Check sheet for the drawn part. Datum: minimum x, y, z corner. Units: mm. A direction names the side the tool comes from. Round coordinates to 2 decimals unless told otherwise and drop trailing zeros. Write each loop counter-clockwise with the first axis right and the second up, starting at its lowest first coordinate (ties: lowest second). Pieces come first, ordered by that corner, then holes. Notation, with made-up numbers: (7.25, 39) - (43.25, 39) arc R17 ccw to (43.25, 63) - close; hole circle Ø3 at (37.5, -4.5). An arc over 180 degrees is marked (long way). Answer as a JSON object with one key per item and string values.
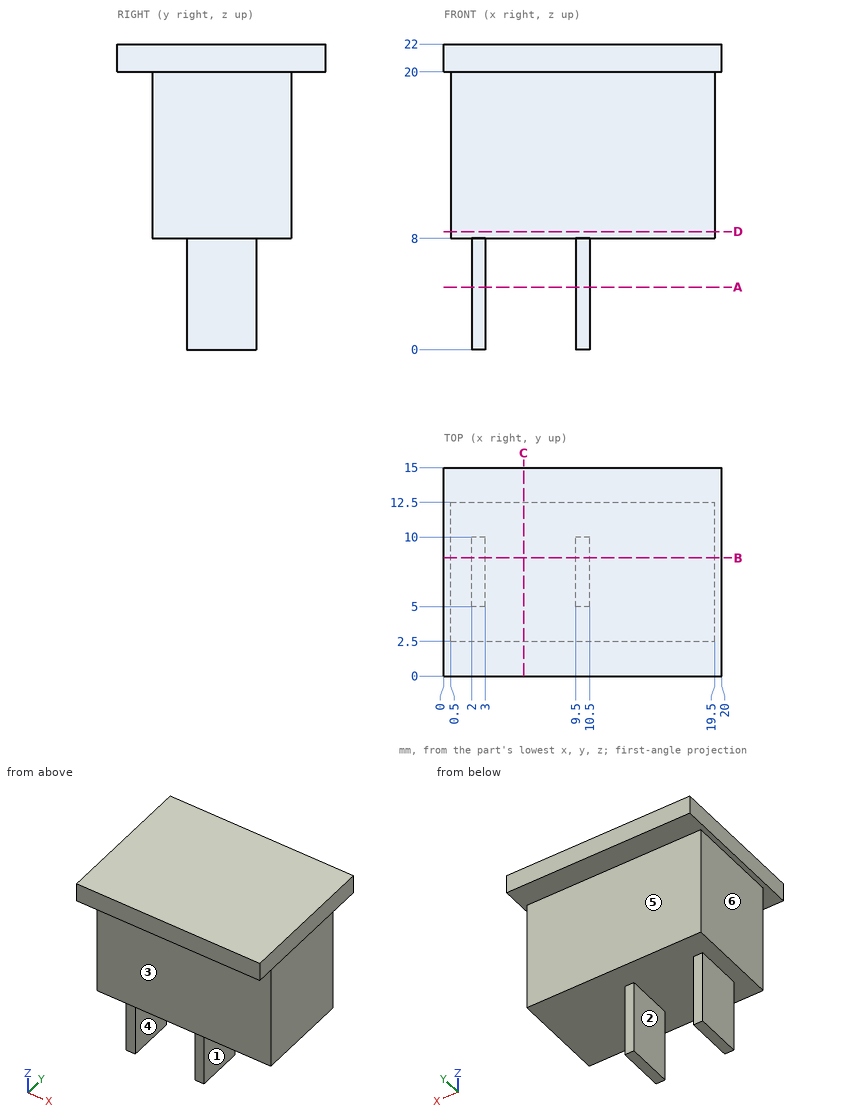
1. Cross-section at A-A (z = 4.5). Record the boundary of the cut face in (x, y), plus the area to 3 significant figures.
Completed:
{"outline": "(2, 5) - (3, 5) - (3, 10) - (2, 10) - close; (9.5, 5) - (10.5, 5) - (10.5, 10) - (9.5, 10) - close", "area": "10.0 mm^2"}
2. Material ranges on probe 1 along X at (y, z) = (8.5, 1.75); probe 2 along Z at (x, y) = (10, 2); probe 3 along X at (y, z) = (12.25, 14), recorded low to high. Write a range as from..to.
Completed:
{"probe 1": "x = 2..3, 9.5..10.5", "probe 2": "z = 20..22", "probe 3": "x = 0.5..19.5"}
3. Go/stop test with flat-tipped pins: pin 1 (0.8 mm diameter, centred on x = 10, z = 5.5, fed in from -Y); pin 2 (4 mm diameter, centred on y = 6.5, z = 4.5, fed in from -X); pin 3 (4 mm diameter, centred on y = 8, z = 5, fed in from +X). Record where each tip stops, or that it passes through.
Completed:
{"pin 1": "stops at y = 5", "pin 2": "stops at x = 2", "pin 3": "stops at x = 10.5"}
4. Cross-section at D-D (z = 8.5). Record the boundary of the cut face in (x, y).
Completed:
{"outline": "(0.5, 2.5) - (19.5, 2.5) - (19.5, 12.5) - (0.5, 12.5) - close"}
5. Access from +Z, -Z, +X, -X, +Y, -Y to the whole of each face (thin tool, end or side, straight path). Record for the marked faces 1, 2 and 3.
Completed:
{"face 1": "-Z, +X, +Y, -Y", "face 2": "-Z, +Y, -Y", "face 3": "-Z, +X, -X, -Y"}
6. Mould release check, pull along X, two halves, no side actions. Record for the marked faces 4, 5 and 6: released by +X, released by -X, zero draft, split by the parting line, or undercut.
Completed:
{"face 4": "undercut", "face 5": "zero draft", "face 6": "released by -X"}
7. Cross-section at B-B (y = 8.5). Record the boundary of the cut face in (x, z), plus the area to 3 significant figures.
Completed:
{"outline": "(0, 20) - (0.5, 20) - (0.5, 8) - (2, 8) - (2, 0) - (3, 0) - (3, 8) - (9.5, 8) - (9.5, 0) - (10.5, 0) - (10.5, 8) - (19.5, 8) - (19.5, 20) - (20, 20) - (20, 22) - (0, 22) - close", "area": "284 mm^2"}
8. Cross-section at C-C (x = 5.75). Record the boundary of the cut face in (y, z).
Completed:
{"outline": "(0, 20) - (2.5, 20) - (2.5, 8) - (12.5, 8) - (12.5, 20) - (15, 20) - (15, 22) - (0, 22) - close"}
